from build123d import *

# Parameters (mm, degrees)
ESQUISSE1_R             = 13
ESQUISSE1_R_2           = 5.5
BOSS_EXTRU_1_DEPTH      = 8
ESQUISSE2_W             = 32.31004566
ESQUISSE2_H             = 49.818141682
ENL_V_MAT_EXTRU_1_DEPTH = 8
ESQUISSE3_R             = 1.5
ENL_V_MAT_EXTRU_2_DEPTH = 8
ESQUISSE4_W             = 21.87123002
ESQUISSE4_H             = 13.833010023
ESQUISSE4_W_2           = 20.432073676
ESQUISSE4_H_2           = 10.309386407
ENL_V_MAT_EXTRU_3_DEPTH = 8
ENL_V_MAT_EXTRU_4_DEPTH = 8
CONG_4_R                = 0.5
ESQUISSE7_W             = 6
ESQUISSE7_H             = 5.75
BOSS_EXTRU_3_DEPTH      = 8
ESQUISSE11_R            = 1.25
ENL_V_MAT_EXTRU_5_DEPTH = 8
CONG_5_R                = 0.5
CONG_6_R                = 1
CONG_7_R                = 0.5


with BuildPart() as part:
    # Esquisse1 → Boss.-Extru.1 (new body)
    with BuildSketch(Plane.XY):
        Circle(ESQUISSE1_R)
        Circle(ESQUISSE1_R_2, mode=Mode.SUBTRACT)
    extrude(amount=BOSS_EXTRU_1_DEPTH)

    # Esquisse2 → Enlèv. mat.-Extru.1 (cut)
    with BuildSketch(Plane.XY.offset(8)):
        with Locations((15.15502283, -0.665904075)):
            Rectangle(ESQUISSE2_W, ESQUISSE2_H)
    extrude(amount=-ENL_V_MAT_EXTRU_1_DEPTH, mode=Mode.SUBTRACT)

    # Esquisse3 → Enlèv. mat.-Extru.2 (cut)
    with BuildSketch(Plane(origin=(-1, 0, 0), x_dir=(0, 0, -1), z_dir=(1, 0, 0))):
        with Locations((-4, 10.461481397)):
            Circle(ESQUISSE3_R)
        with Locations((-4, -10.461481397)):
            Circle(ESQUISSE3_R)
    extrude(amount=-ENL_V_MAT_EXTRU_2_DEPTH, mode=Mode.SUBTRACT)

    # Esquisse4 → Enlèv. mat.-Extru.3 (cut)
    with BuildSketch(Plane.XY.offset(8)):
        with Locations((-17.93561501, 14.127986408)):
            Rectangle(ESQUISSE4_W, ESQUISSE4_H)
        with Locations((-17.216036838, -12.366174601)):
            Rectangle(ESQUISSE4_W_2, ESQUISSE4_H_2)
    extrude(amount=-ENL_V_MAT_EXTRU_3_DEPTH, mode=Mode.SUBTRACT)

    # Esquisse6 → Enlèv. mat.-Extru.4 (cut)
    with BuildSketch(Plane.XY.offset(8)):
        with BuildLine():
            Line((-16.733633374, -12.244867556), (-8.177661786, -8.782132299))
            ThreePointArc((-8.177661786, -8.782132299), (-11.997254104, 0.256698201), (-7.794537354, 9.123880065))
            Line((-7.794537354, 9.123880065), (-13.177897042, 8.696922023))
            ThreePointArc((-13.177897042, 8.696922023), (-19.765548318, -0.95731283), (-16.733633374, -12.244867556))
        make_face()
    extrude(amount=-ENL_V_MAT_EXTRU_4_DEPTH, mode=Mode.SUBTRACT)

    # Congé4
    cong_4_edges = [part.edges().sort_by_distance(p)[0] for p in [
        (-9.591378215, 7.211481397, 4),
        (-9.591378215, -7.211481397, 4),
    ]]
    fillet(cong_4_edges, radius=CONG_4_R)

    # Esquisse7 → Boss.-Extru.3 (add)
    with BuildSketch(Plane(origin=(0, 0, 0), x_dir=(-1, 0, 0), z_dir=(0, 0, -1))):
        with Locations((4, 10.086481397)):
            Rectangle(ESQUISSE7_W, ESQUISSE7_H)
        with Locations((4, -10.086481397)):
            Rectangle(ESQUISSE7_W, ESQUISSE7_H)
    extrude(amount=-BOSS_EXTRU_3_DEPTH)

    # Esquisse11 → Enlèv. mat.-Extru.5 (cut)
    with BuildSketch(Plane(origin=(-1, 0, 0), x_dir=(0, 0, -1), z_dir=(1, 0, 0))):
        with Locations((-4, 10.461481397)):
            Circle(ESQUISSE11_R)
        with Locations((-4, -10.461481397)):
            Circle(ESQUISSE11_R)
    extrude(amount=-ENL_V_MAT_EXTRU_5_DEPTH, mode=Mode.SUBTRACT)

    # Congé5
    cong_5_edges = [part.edges().sort_by_distance(p)[0] for p in [
        (-7, 12.961481397, 4),
        (-7, -12.961481397, 4),
    ]]
    fillet(cong_5_edges, radius=CONG_5_R)

    # Congé6
    cong_6_edges = [part.edges().sort_by_distance(p)[0] for p in [
        (-7, 7.211481397, 4),
        (-7, -7.211481397, 4),
    ]]
    fillet(cong_6_edges, radius=CONG_6_R)

    # Congé7
    cong_7_edges = [part.edges().sort_by_distance(p)[0] for p in [
        (-1, 12.961481397, 4),
        (-1, -12.961481397, 4),
    ]]
    fillet(cong_7_edges, radius=CONG_7_R)


solid = part.part
Geometry: final body of the model. Coordinates: model frame, mm. A direction names the side the tool comes from. Coordinates: 2 decimals unless noted, no trailing zeros. Write each loop counter-clockwise with the first axis right and the second up, starting at its lowest first coordinate (ties: lowest second). Pieces come first, ordered by that corner, then holes. Notation, with made-up numbers: (31.25, 21.25) - (71.25, 21.25) arc R37 cw to (71.25, 57.25) - close; hole circle Ø10 at (74.5, -22). An arc over 180 degrees is marked (long way). Return JSON: item names as keys, results as strings.
Item 1: Section query D-D (z = 5.75). Output: boundary loops of the cut face in (x, y).
Completed:
{"outline": "(-9.74, -7) arc R0.5 ccw to (-9.34, -7.21) - (-8, -7.21) arc R1 cw to (-7, -8.21) - (-7, -12.46) arc R0.5 ccw to (-6.5, -12.96) - (-1.5, -12.96) arc R0.5 ccw to (-1, -12.46) - (-1, -5.41) arc R5.5 cw to (-1, 5.41) - (-1, 12.46) arc R0.5 ccw to (-1.5, 12.96) - (-6.5, 12.96) arc R0.5 ccw to (-7, 12.46) - (-7, 8.21) arc R1 cw to (-8, 7.21) - (-9.34, 7.21) arc R0.5 ccw to (-9.74, 7) arc R12 ccw to start"}
Item 2: Pin query (flat end, axial travel): pin 1 Ø1.5 at (y, z) = (10, 5.5) entering from -X; pin 2 Ø4 at (x, z) = (-10, 5.5) entering from +Y; pin 3 Ø3 at (x, y) = (-11, -9.5) entering from -Z; pin 4 Ø1.5 at (y, z) = (0, 4.5) entering from +X. Return the tip coordinate at first contact, or that it passes through.
Completed:
{"pin 1": "stops at x = -7", "pin 2": "stops at y = 7.21", "pin 3": "passes through", "pin 4": "stops at x = -5.45"}
Item 3: Section query B-B (y = -9.5). Output: boundary loops of the cut face in (x, z), and give its area (3 significant figures).
Completed:
{"outline": "(-7, 0) - (-1, 0) - (-1, 3.2) - (-7, 3.2) - close; (-7, 4.8) - (-1, 4.8) - (-1, 8) - (-7, 8) - close", "area": "38.4 mm2"}
Item 4: Line query: L1, parallel to Y at x = -5.8, z = 4; L2, parallel to Y at x = -2.5, z = 3; L3, parallel to Y at x = -3.25, z = 4.5. Output: solid intervals per line, ascending.
Completed:
{"L1": "y = -12.96 to -11.71, -9.21 to 9.21, 11.71 to 12.96", "L2": "y = -12.96 to -11.21, -9.71 to -4.9, 4.9 to 9.71, 11.21 to 12.96", "L3": "y = -12.96 to -11.61, -9.32 to -4.44, 4.44 to 9.32, 11.61 to 12.96"}
Item 5: Section query C-C (x = -6.75). Output: boundary loops of the cut face in (y, z).
Completed:
{"outline": "(-12.89, 0) - (12.89, 0) - (12.89, 8) - (-12.89, 8) - close; hole circle Ø2.5 at (-10.46, 4); hole circle Ø2.5 at (10.46, 4)"}
Item 6: Pull-direction query (Y, two-part tool) for faces 1 (the face through (-7.3, 7.5, 3.9)), 2 (the face through (-5.5, 0.1, 3.9)), 3 (the face through (-7, 0, 8)); classes: +Y half, -Y half, draft (parallel to the pull), parting line (faces both ways), or undercut.
Completed:
{"face 1": "+Y half", "face 2": "undercut", "face 3": "draft"}
Item 7: Reachability of faces 4 (the face through (-1, 9, 4)), 5 (the face through (-7, 9, 5)), 6 (the face through (-7, -9, 5)) from +Z, -Z, +X, -X, +Y, -Y: full face, straight path, thin tool, end or side. Return the list, or none.
Completed:
{"face 4": "+Z, -Z, +X, +Y, -Y", "face 5": "+Z, -Z, -X, +Y", "face 6": "+Z, -Z, -X, -Y"}
Item 8: Section query A-A (z = 4). Output: boundary loops of the cut face in (x, y), and give its area (3 significant figures).
Completed:
{"outline": "(-9.74, -7) arc R0.5 ccw to (-9.34, -7.21) - (-8, -7.21) arc R1 cw to (-7, -8.21) - (-7, -9.21) - (-1, -9.21) - (-1, -5.41) arc R5.5 cw to (-1, 5.41) - (-1, 9.21) - (-7, 9.21) - (-7, 8.21) arc R1 cw to (-8, 7.21) - (-9.34, 7.21) arc R0.5 ccw to (-9.74, 7) arc R12 ccw to start; (-7, -12.46) arc R0.5 ccw to (-6.5, -12.96) - (-1.5, -12.96) arc R0.5 ccw to (-1, -12.46) - (-1, -11.71) - (-7, -11.71) - close; (-7, 11.71) - (-1, 11.71) - (-1, 12.46) arc R0.5 ccw to (-1.5, 12.96) - (-6.5, 12.96) arc R0.5 ccw to (-7, 12.46) - close", "area": "150 mm2"}
